Build history of the part. All positions in model axes, mm. A direction names the side the tool comes from. Give positions to 0.01 mm unless a question says otherwise; leave off trailing zeros. Write each loop counter-clockwise with the first axis right and the second up, starting at its lowest first coordinate (ties: lowest second). Pieces come first, ordered by that corner, then holes. Notation, with made-up numbers: (-1, 83.25) -> (46, 83.25) arc R36 cw to (46, 120.25) -> close; hole circle Ø5 at (-4, 40). An arc over 180 degrees is marked (long way). One line per question, with ' | ' between items. Start each with the question number.
(1) Pin check, flat tips, straight feed: P1, Ø4, axis at x = 47.5, z = -2.5, coming from the +Y side; P2, Ø1.2, axis at y = 2.5, z = -5.5, coming from the +X side; P3, Ø3, axis at x = 42, z = -33.5, coming from the +Y side; P4, Ø1.6, axis at y = 0.5, z = -24, coming from the +X side. Stop position of each tip, or through.
(2) Tool access for faces 1 (the flat face through (25, 3, -16.667)), 2 (the flat face through (16.667, 3, -8)), 3 (the flat face through (33.333, 3, -8)), 4 (the flat face through (47.5, 1, -25)): list every direction of +Z, -Z, +X, -X, +Y, -Y with a clear straight run to the whole face (end or side of a thin tool).
(3) Band-saw the part on B-B, the plane y = 4.05. Give the cut face in (x, z), and give its area (3 significant figures).
(4) Pull direction Z, two halves, no side cores. Call faces 5 (the flat face through (46, 1, -50)), 6 (the cylindrical face through (46.161, 0.74, -49.246)), 7 (the flat face through (50, 1, -4)): released by +Z, released by -Z, zero draft, split by the parting line, or undercut.
(5) Band-saw the part on A-A, the plane z = -2.5. Give the cut face in (x, y), and give its area (3 significant figures).
(6) Drill centre lines: probe 1 along X at (y, z) = (1.15, -2.5); probe 2 along Z at (x, y) = (4, 0.65); probe 3 along Z at (x, y) = (33, 3.35). Where is each one in solid material? Low to high. Write a range as from..to.
(7) Band-saw the part on C-C, the plane x = 38. Give the cut face in (y, z), and give its area (4 significant figures).
from build123d import *

# Parameters (mm, degrees)
SKETCH1_W           = 50
SKETCH1_H           = 50
SKETCH1_R           = 2.2
BOSS_EXTRUDE1_DEPTH = 1.5
SKETCH3_W           = 2.555545098
SKETCH3_H           = 35
SKETCH3_W_2         = 2.5
SKETCH3_W_3         = 35
SKETCH3_H_2         = 2.5
CUT_EXTRUDE1_DEPTH  = 1.5
FILLET8_R           = 1
SKETCH4_W           = 16.6666
SKETCH4_H           = 16.6666
BOSS_EXTRUDE2_DEPTH = 4


with BuildPart() as part:
    # Sketch1 → Boss-Extrude1 (new body)
    with BuildSketch(Plane(origin=(0, 0, 0), x_dir=(1, 0, 0), z_dir=(0, 1, 0))):
        with Locations((25, 25)):
            Rectangle(SKETCH1_W, SKETCH1_H)
        with Locations(Location((2.555545098, 47.5, 0), (0, 0, 270))):
            Circle(SKETCH1_R, mode=Mode.SUBTRACT)
        with Locations(Location((47.5, 47.5, 0), (0, 0, 270))):
            Circle(SKETCH1_R, mode=Mode.SUBTRACT)
        with Locations(Location((2.5, 2.5, 0), (0, 0, 270))):
            Circle(SKETCH1_R, mode=Mode.SUBTRACT)
        with Locations(Location((47.5, 2.5, 0), (0, 0, 270))):
            Circle(SKETCH1_R, mode=Mode.SUBTRACT)
    extrude(amount=BOSS_EXTRUDE1_DEPTH)

    # Sketch3 → Cut-Extrude1 (cut)
    with BuildSketch(Plane(origin=(0, 0, 0), x_dir=(1, 0, 0), z_dir=(0, 1, 0))):
        with Locations((1.277772549, 25)):
            Rectangle(SKETCH3_W, SKETCH3_H)
        with Locations((48.75, 25)):
            Rectangle(SKETCH3_W_2, SKETCH3_H)
        with Locations((25, 48.75)):
            Rectangle(SKETCH3_W_3, SKETCH3_H_2)
    extrude(amount=CUT_EXTRUDE1_DEPTH, mode=Mode.SUBTRACT)

    # Fillet8
    fillet8_edges = [part.edges().sort_by_distance(p)[0] for p in [
        (0, 0.75, -7.5),
        (2.555545098, 0.75, -7.5),
        (2.555545098, 0.75, -42.5),
        (0, 0.75, -42.5),
        (47.5, 0.75, -7.5),
        (50, 0.75, -7.5),
        (50, 0.75, -42.5),
        (47.5, 0.75, -42.5),
        (7.5, 0.75, -47.5),
        (42.5, 0.75, -47.5),
        (42.5, 0.75, -50),
        (7.5, 0.75, -50),
        (0, 0.75, -50),
        (50, 0.75, -50),
        (50, 0.75, 0),
        (0, 0.75, 0),
    ]]
    fillet(fillet8_edges, radius=FILLET8_R)

    # Sketch4 → Boss-Extrude2 (add)
    with BuildSketch(Plane(origin=(0, 1.5, 0), x_dir=(1, 0, 0), z_dir=(0, 1, 0))):
        with Locations((25, 8.3333)):
            Rectangle(SKETCH4_W, SKETCH4_H)
    extrude(amount=BOSS_EXTRUDE2_DEPTH)


solid = part.part
Results:
1) P1: passes through | P2: stops at x = 33.33 | P3: stops at y = 1.5 | P4: stops at x = 47.5
2) face 1: -Z, +X, -X, +Y | face 2: +Z, -Z, -X, +Y | face 3: +Z, -Z, +X, +Y | face 4: +X, +Y, -Y
3) outline: (16.67, -16.67) -> (33.33, -16.67) -> (33.33, 0) -> (16.67, 0) -> close | area: 278 mm²
4) face 5: released by -Z | face 6: undercut | face 7: zero draft
5) outline: (0, 0) -> (0.3, 0) -> (0.3, 1.5) -> (0, 1.5) -> close; (4.7, 0) -> (45.3, 0) -> (45.3, 1.5) -> (33.33, 1.5) -> (33.33, 5.5) -> (16.67, 5.5) -> (16.67, 1.5) -> (4.7, 1.5) -> close; (49.7, 0) -> (50, 0) -> (50, 1.5) -> (49.7, 1.5) -> close | area: 128 mm²
6) probe 1: x = 0..0.3, 4.7..45.3, 49.7..50 | probe 2: z = -50..-49.16, -45.84..-4.11, -0.89..0 | probe 3: z = -16.67..0
7) outline: (0, -47.5) -> (1.5, -47.5) -> (1.5, 0) -> (0, 0) -> close | area: 71.25 mm²
